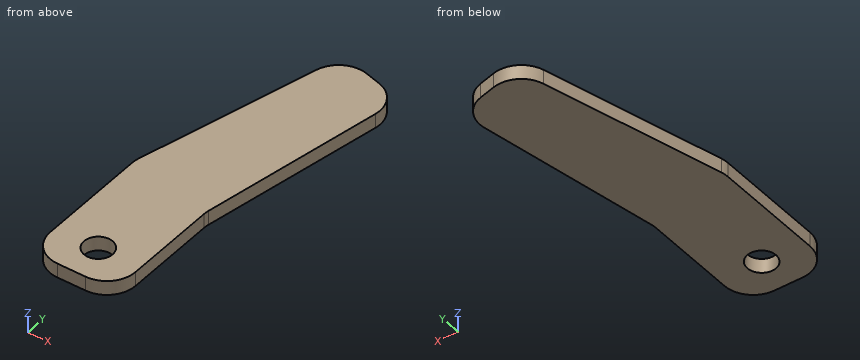
from build123d import *

# Parameters (mm, degrees)
SKETCH1_R           = 1
BOSS_EXTRUDE1_DEPTH = 1
FILLET1_R           = 2
FILLET2_R           = 2
FILLET3_R           = 2
FILLET4_R           = 2
FILLET5_R           = 2
FILLET6_R           = 2


with BuildPart() as part:
    # Sketch1 → Boss-Extrude1 (new body)
    with BuildSketch(Plane.XY):
        Polygon((0, 10), (3.882285677, 24.488887394), (8.711914808, 23.194792169), (5.965925826, 8.639463055), (5.965925826, 8.027846959), (5.965925826, 0), (0, 0), align=None)
        with Locations((2.999793512, 2.5)):
            Circle(SKETCH1_R, mode=Mode.SUBTRACT)
    extrude(amount=BOSS_EXTRUDE1_DEPTH)

    # Fillet1
    fillet1_edges = [part.edges().sort_by_distance(p)[0] for p in [
        (5.965925826, 0, 0.5),
    ]]
    fillet(fillet1_edges, radius=FILLET1_R)

    # Fillet2
    fillet2_edges = [part.edges().sort_by_distance(p)[0] for p in [
        (0, 0, 0.5),
    ]]
    fillet(fillet2_edges, radius=FILLET2_R)

    # Fillet3
    fillet3_edges = [part.edges().sort_by_distance(p)[0] for p in [
        (8.711914808, 23.194792169, 0.5),
    ]]
    fillet(fillet3_edges, radius=FILLET3_R)

    # Fillet4
    fillet4_edges = [part.edges().sort_by_distance(p)[0] for p in [
        (3.882285677, 24.488887394, 0.5),
    ]]
    fillet(fillet4_edges, radius=FILLET4_R)

    # Fillet5
    fillet5_edges = [part.edges().sort_by_distance(p)[0] for p in [
        (0, 10, 0.5),
    ]]
    fillet(fillet5_edges, radius=FILLET5_R)

    # Fillet6
    fillet6_edges = [part.edges().sort_by_distance(p)[0] for p in [
        (5.965925826, 8.639463055, 0.5),
    ]]
    fillet(fillet6_edges, radius=FILLET6_R)


solid = part.part
Read the model definition and answer for the solid it produces. Units are mm, in the model's axes. Coordinates: 2 decimals unless noted, no trailing zeros. Write each loop counter-clockwise with the first axis right and the second up, starting at its lowest first coordinate (ties: lowest second). Pieces come first, ordered by that corner, then holes. Notation, with made-up numbers: (-5, 3) - (27, 3) arc R17 cw to (27, 11) - close; hole circle Ø10 at (62, 37). An arc over 180 degrees is marked (long way). One line per question, with ' | ' between items.
Q1. Consider L1, parallel to Y at x = 4.25, z = 0.05; L2, parallel to Y at x = 5.75, z = 0.25; L3, parallel to X at y = 1.25, z = 0.45. Determine where each line is inside the solid, lowest interval first. Write a range as [from, to].
Result set:
L1: [0.02, 23.74] | L2: [1.1, 23.99] | L3: [0.15, 5.82]
Q2. Find section A-A, the plane y = 2.5. Write down the section's boundary in (x, z), plus the area to 3 significant figures.
Result set:
outline: (0, 0) - (2, 0) - (2, 1) - (0, 1) - close; (4, 0) - (5.97, 0) - (5.97, 1) - (4, 1) - close | area: 3.97 mm^2
Q3. Find section C-C, the plane x = 2.25. Write down the section's boundary in (y, z).
Result set:
outline: (0, 0) - (1.84, 0) - (1.84, 1) - (0, 1) - close; (3.16, 0) - (18.4, 0) - (18.4, 1) - (3.16, 1) - close
Q4. Find section D-D, the plane y = 6.75. Write down the section's boundary in (x, z), plus the area to 3 significant figures.
Result set:
outline: (0, 0) - (5.97, 0) - (5.97, 1) - (0, 1) - close | area: 5.97 mm^2
Q5. Find section B-B, the plane z = 0.25. Write down the section's boundary in (x, y), plus the area to 3 significant figures.
Result set:
outline: (0, 2) arc R2 ccw to (2, 0) - (3.97, 0) arc R2 ccw to (5.97, 2) - (5.97, 8.45) arc R2 cw to (6, 8.82) - (8.37, 21.37) arc R2 ccw to (6.92, 23.67) - (5.81, 23.97) arc R2 ccw to (3.36, 22.56) - (0.07, 10.25) arc R2 ccw to (0, 9.74) - close; hole circle Ø2 at (3, 2.5) | area: 132 mm^2
